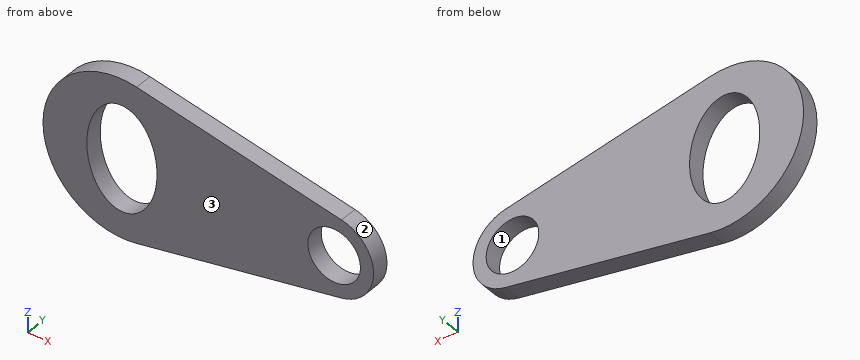
```python
from build123d import *

# Parameters (mm, degrees)
SKETCH1_R           = 15
SKETCH1_RX          = 30
SKETCH1_RY          = 20
BOSS_EXTRUDE1_DEPTH = 10


with BuildPart() as part:
    # Sketch1 → Boss-Extrude1 (new body)
    with BuildSketch(Plane(origin=(0, 0, 0), x_dir=(1, 0, 0), z_dir=(0, 1, 0))):
        with BuildLine():
            Line((-34.444842367, 44.214814759), (82.343924077, 22.10740738))
            ThreePointArc((82.343924077, 22.10740738), (100.659125522, 0), (82.343924077, -22.10740738))
            Line((82.343924077, -22.10740738), (-34.444842367, -44.214814759))
            ThreePointArc((-34.444842367, -44.214814759), (-87.814439477, 0), (-34.444842367, 44.214814759))
        make_face()
        with Locations(Location((78.159125522, 0, 0), (0, 0, 270))):
            Circle(SKETCH1_R, mode=Mode.SUBTRACT)
        with Locations(Location((-42.814439477, 0), (0, 0, 90))):
            Ellipse(SKETCH1_RX, SKETCH1_RY, mode=Mode.SUBTRACT)
    extrude(amount=BOSS_EXTRUDE1_DEPTH)


solid = part.part
```
Work out the finished part from the listing and answer in its coordinate system (mm). Face numbers are marked on the shaded views. Coordinates: 2 decimals unless noted, no trailing zeros. Loops run counter-clockwise (first coordinate to the right, second up) from the corner with the lowest first, then second, coordinate; pieces in that order, holes last. Notation, with made-up numbers: M 65,-13 L 85,-13 A12 cw 85,-2 Z; hole C -15.5,41.5 d1. An arc over 180 degrees is marked long. Use CSV: the item, a comma, the result in double quotes. Start each with the question number.
(1) Find section D-D, the plane x = 0.5. Give the vertices of the cut face in (y, z), then the cut area to 3 significant figures.
(2) Consider line 1 (X direction, y = 2.5, z = 12); line 2 (Z direction, x = 81, y = 0.5); line 3 (Z direction, x = 68, y = 1.25). Determine where each line is inside the solid, lowest interval first.
(3) Given pin 1 Ø6 at (x, y) = (54.5, 6.5) entering from +Z; pin 2 Ø1 at (y, z) = (4, -17.5) entering from +X; pin 3 Ø5 at (x, y) = (56, 5) entering from -Z, each flat-ended and moving along its own axis, determine where each tip first touches the part or whether it passes through.
(4) Find section A-A, the plane z = 0. State how many separate pieces and enclosed holes the cut face has, then the cut area to 3 significant figures.
(5) For a pull along X with two mould halves and no side action, classify the marked faces 1, 2 and 3 as +X half, -X half, draft (parallel to the pull), parting line (faces both ways), or undercut.
Recorded:
1,outline,"M 0,-37.6 L 10,-37.6 L 10,37.6 L 0,37.6 Z"
1,area,"752 mm^2"
2,line 1,"x = -86.18 to -61.14, -24.48 to 69.16, 87.16 to 97.19"
2,line 2,"z = -22.36 to -14.73, 14.73 to 22.36"
2,line 3,"z = -24.82 to -11.04, 11.04 to 24.82"
3,pin 1,"stops at z = 27.95"
3,pin 2,"stops at x = 92.9"
3,pin 3,"stops at z = -27.57"
4,separate pieces,"3"
4,enclosed holes,"0"
4,area,"1,180 mm^2"
5,face 1,"undercut"
5,face 2,"+X half"
5,face 3,"draft"
